from build123d import *

# Parameters (mm, degrees)
SKETCH5_W                = 30
SKETCH5_H                = 100
BOSS_EXTRUDE2_DEPTH      = 7.1
SKETCH7_W                = 6.895
SKETCH7_H                = 20
SKETCH7_H_2              = 21
CUT_EXTRUDE2_DEPTH       = 140.379819119
SKETCH8_W                = 60
SKETCH8_H                = 5
SPLIT2_SURFACE_1_BACK    = 107.419
SPLIT2_SURFACE_1_DEPTH   = 214.838
SKETCH10_R               = 2.5
CUT_EXTRUDE5_DEPTH       = 20
CUT_EXTRUDE5_DEPTH_BACK  = 67
CUT_EXTRUDE7_DEPTH       = 140.461200617
CUT_EXTRUDE7_DEPTH_BACK  = 140.461200617
SKETCH41_W               = 15.603241914
SKETCH41_H               = 21
CUT_EXTRUDE9_DEPTH       = 140.461200617
CUT_EXTRUDE9_DEPTH_BACK  = 140.461200617
SCALE1_SCALE             = 0.35
SKETCH46_W               = 2
SKETCH46_H               = 3
CUT_EXTRUDE10_DEPTH      = 111.657018213
CUT_EXTRUDE10_DEPTH_BACK = 111.657018213
BOSS_EXTRUDE3_REACH      = 70.762
SKETCH47_W               = 0.5
SKETCH47_H               = 2.485


with BuildPart() as part:
    # Sketch5 → Boss-Extrude2 (new body)
    with BuildSketch(Plane(origin=(0, 0, 0), x_dir=(1, 0, 0), z_dir=(0, 1, 0))):
        with Locations((81.879400831, -49.953517558)):
            Rectangle(SKETCH5_W, SKETCH5_H)
    extrude(amount=BOSS_EXTRUDE2_DEPTH)

    # Sketch7 → Cut-Extrude2 (cut, through all)
    with BuildSketch(Plane(origin=(0, 7.1, 0), x_dir=(1, 0, 0), z_dir=(0, 1, 0))):
        with Locations((70.326900831, -9.953517558)):
            Rectangle(SKETCH7_W, SKETCH7_H)
        with Locations((70.326900831, -49.953517558)):
            Rectangle(SKETCH7_W, SKETCH7_H_2)
        with Locations((70.326900831, -89.953517558)):
            Rectangle(SKETCH7_W, SKETCH7_H)
    extrude(amount=-CUT_EXTRUDE2_DEPTH, mode=Mode.SUBTRACT)

    # Sketch8 → Revolve-Thin2 (revolve)
    with BuildSketch(Plane.ZY.offset(-66.879400831), mode=Mode.PRIVATE) as revolve_thin2_sk:
        with Locations((49.953517558, 6.05)):
            Rectangle(SKETCH8_W, SKETCH8_H)
    revolve(revolve_thin2_sk.sketch.rotate(Axis((66.879400831, 3.55, 19.953517558), (0, 0, 1)), 315.234915329), axis=Axis((66.879400831, 3.55, 19.953517558), (0, 0, 1)))

    # Split2: cut with a surface, the side behind it stays
    # Split2 surface: a surface, the sketch's curves swept straight by 214.838 mm
    with BuildLine(Plane(origin=(0, 7.1, 0), x_dir=(1, 0, 0), z_dir=(0, 1, 0)).offset(-SPLIT2_SURFACE_1_BACK), mode=Mode.PRIVATE) as split2_surface_1_path:
        Line((71.879400831, -39.453517558), (61.879400831, -39.453517558))
        Line((61.879400831, -39.453517558), (61.879400831, -59.953517558))
        Line((61.879400831, -59.953517558), (71.879400831, -59.953517558))
        Line((71.879400831, -59.953517558), (71.879400831, -39.453517558))
    split2_surface_1 = Shell.extrude(split2_surface_1_path.wire(), (0 * SPLIT2_SURFACE_1_DEPTH, 1 * SPLIT2_SURFACE_1_DEPTH, 0 * SPLIT2_SURFACE_1_DEPTH))
    split(bisect_by=split2_surface_1, keep=Keep.BOTTOM)

    # Sketch10 → Cut-Extrude5 (cut, two sides)
    with BuildSketch(Plane.XY.offset(79.953517558)) as cut_extrude5_sk:
        with Locations(Location((66.879400831, 3.55, 0), (0, 0, 180))):
            Circle(SKETCH10_R)
    extrude(amount=CUT_EXTRUDE5_DEPTH, mode=Mode.SUBTRACT)
    extrude(cut_extrude5_sk.sketch, amount=-CUT_EXTRUDE5_DEPTH_BACK, mode=Mode.SUBTRACT)

    # Sketch36 → Cut-Extrude7 (cut, two sides)
    with BuildSketch(Plane(origin=(0, 0, 0), x_dir=(1, 0, 0), z_dir=(0, 1, 0))) as cut_extrude7_sk:
        Polygon((62.879400831, -39.453517558), (61.879400831, -38.753517558), (61.879400831, -39.453517558), align=None)
        Polygon((61.879400831, -59.953517558), (62.879400831, -59.953517558), (61.879400831, -60.653517558), align=None)
        Polygon((62.879400831, -79.953517558), (61.879400831, -79.253517558), (61.879400831, -79.953517558), align=None)
        Polygon((61.879400831, -19.953517558), (62.879400831, -19.953517558), (61.879400831, -20.653517558), align=None)
    extrude(amount=CUT_EXTRUDE7_DEPTH, mode=Mode.SUBTRACT)
    extrude(cut_extrude7_sk.sketch, amount=-CUT_EXTRUDE7_DEPTH_BACK, mode=Mode.SUBTRACT)

    # Sketch41 → Cut-Extrude9 (cut, two sides)
    with BuildSketch(Plane(origin=(0, 7.1, 0), x_dir=(1, 0, 0), z_dir=(0, 1, 0))) as cut_extrude9_sk:
        with Locations((65.972779874, -49.953517558)):
            Rectangle(SKETCH41_W, SKETCH41_H)
    extrude(amount=CUT_EXTRUDE9_DEPTH, mode=Mode.SUBTRACT)
    extrude(cut_extrude9_sk.sketch, amount=-CUT_EXTRUDE9_DEPTH_BACK, mode=Mode.SUBTRACT)


with BuildPart() as part_1:
    # Scale1: scaled about (82.710750678, 3.55, 49.954128315)
    add(part.part.scale(SCALE1_SCALE).moved(Location((53.761987941, 2.3075, 32.470183405))))

    # Sketch46 → Cut-Extrude10 (cut, two sides)
    with BuildSketch(Plane(origin=(0, 4.792503371, 0), x_dir=(1, 0, 0), z_dir=(0, 1, 0))) as cut_extrude10_sk:
        with Locations((86.669801184, -43.953922739)):
            Rectangle(SKETCH46_W, SKETCH46_H)
        with Locations((86.669801184, -55.953922739)):
            Rectangle(SKETCH46_W, SKETCH46_H)
    extrude(amount=CUT_EXTRUDE10_DEPTH, mode=Mode.SUBTRACT)
    extrude(cut_extrude10_sk.sketch, amount=-CUT_EXTRUDE10_DEPTH_BACK, mode=Mode.SUBTRACT)

    # Sketch47 → Boss-Extrude3 (add, up to next)
    with BuildSketch(Plane(origin=(87.669801184, 0, 0), x_dir=(0, 0, -1), z_dir=(1, 0, 0)), mode=Mode.PRIVATE) as boss_extrude3_sk1:
        with Locations((-57.203922739, 3.550003371)):
            Rectangle(SKETCH47_W, SKETCH47_H)
    boss_extrude3_tool1 = extrude(boss_extrude3_sk1.sketch, amount=-BOSS_EXTRUDE3_REACH, mode=Mode.PRIVATE) - part_1.part
    # Sketch47 → Boss-Extrude3 (add, up to next)
    with BuildSketch(Plane(origin=(87.669801184, 0, 0), x_dir=(0, 0, -1), z_dir=(1, 0, 0)), mode=Mode.PRIVATE) as boss_extrude3_sk2:
        with Locations((-45.203922739, 3.550003371)):
            Rectangle(SKETCH47_W, SKETCH47_H)
    boss_extrude3_tool2 = extrude(boss_extrude3_sk2.sketch, amount=-BOSS_EXTRUDE3_REACH, mode=Mode.PRIVATE) - part_1.part
    add(boss_extrude3_tool1.solids().sort_by_distance((87.669801, 3.550003, 57.203923))[0])
    add(boss_extrude3_tool2.solids().sort_by_distance((87.669801, 3.550003, 45.203923))[0])


solid = part_1.part
Check sheet for the modelled part. Datum: model origin and axes. Units: mm. A direction names the side the tool comes from. Coordinates: 2 decimals unless noted, no trailing zeros. Loops run counter-clockwise (first coordinate to the right, second up) from the corner with the lowest first, then second, coordinate; pieces in that order, holes last. Notation, with made-up numbers: (-4.75, -12) -> (27.25, -12) arc R18 ccw to (27.25, 1) -> close; hole circle Ø4 at (-38, -9). An arc over 180 degrees is marked (long way). Answer in a Markdown table with one row per item.
1. Sectioned sample at D-D, the plane x = 77.25. Record the boundary of the cut face in (y, z).
Check values:
| item | result |
|---|---|
| outline | (1.8, 39.45) -> (2.68, 39.45) -> (2.68, 46.28) -> (1.8, 46.28) -> close; (1.8, 53.63) -> (2.68, 53.63) -> (2.68, 60.45) -> (1.8, 60.45) -> close; (4.42, 39.45) -> (5.3, 39.45) -> (5.3, 46.28) -> (4.42, 46.28) -> close; (4.42, 53.63) -> (5.3, 53.63) -> (5.3, 60.45) -> (4.42, 60.45) -> close |
2. Release check for a two-part mould opening along Z. For faces 6 (the face through (78.1, 4, 39.454)), 7 (the face through (78.4, 3.6, 60.454)), 8 (the face through (85.67, 4, 44)), 9 (the face through (79.583, 4, 64)) record: released by +Z, released by -Z, zero draft, split by the parting line, or undercut.
Check values:
| item | result |
|---|---|
| face 6 | released by -Z |
| face 7 | released by +Z |
| face 8 | undercut |
| face 9 | zero draft |
3. Access from +Z, -Z, +X, -X, +Y, -Y to the whole of each face (thin tool, end or side, straight path). Record for faces 1 (the face through (87, 4, 42.454)), 2 (the face through (87.67, 4, 63)), 3 (the face through (79.583, 4, 36)), 4 (the face through (78.1, 3.1, 46.279)), 5 (the face through (83, 4.792, 62)).
Check values:
| item | result |
|---|---|
| face 1 | +X, +Y, -Y |
| face 2 | +Z, -Z, +X, +Y, -Y |
| face 3 | -Z, -X, +Y, -Y |
| face 4 | -X, +Y, -Y |
| face 5 | +Z, -Z, +X, +Y |
4. Material ranges on line 1 along Z through (x, y) = (87, 3.3); line 2 along X through (y, z) = (3.55, 56.5); line 3 along Z through (x, y) = (76.75, 2.35), recorded low to high. Write a range as [from, to].
Check values:
| item | result |
|---|---|
| line 1 | z = [32.45, 42.45], [44.95, 54.45], [56.95, 67.45] |
| line 2 | x = [75.42, 76.29], [78.04, 85.67] |
| line 3 | z = [39.45, 46.28], [53.63, 60.45] |
5. Sectioned sample at A-A, the plane x = 87.25. Give the number of separate pieces and of enclosed holes in the cut face, then the cut area to 4 significant figures.
Check values:
| item | result |
|---|---|
| separate pieces | 3 |
| enclosed holes | 0 |
| area | 74.55 mm2 |
6. Go/stop test with flat-tipped pins: pin 1 (0.7 mm diameter, centred on y = 3.5, z = 50, fed in from -X); pin 2 (1 mm diameter, centred on x = 78, y = 4, fed in from +Z); pin 3 (1.5 mm diameter, centred on x = 84.5, z = 62, fed in from -Y); pin 4 (1.2 mm diameter, centred on y = 3, z = 56.5, fed in from +X). Record where each tip stops, or that it passes through.
Check values:
| item | result |
|---|---|
| pin 1 | stops at x = 79.58 |
| pin 2 | stops at z = 60.45 |
| pin 3 | stops at y = 2.31 |
| pin 4 | stops at x = 87.67 |
